```python
from build123d import *

# Parameters (mm, degrees)
PAD025_DEPTH    = 1
SKETCH038_W     = 8.1
SKETCH038_H     = 3.05
SKETCH038_W_2   = 3.05
SKETCH038_H_2   = 8.1
POCKET013_DEPTH = 0.5
POCKET014_DEPTH = 0.25
POCKET015_DEPTH = 0.25
SKETCH041_W     = 8
SKETCH041_H     = 3
SKETCH041_W_2   = 3
SKETCH041_H_2   = 8
PAD026_DEPTH    = 0.5


with BuildPart() as part:
    # Sketch037 (on Face2 of Binder012) → Pad025 (new body)
    with BuildSketch(Plane(origin=(0, 0, -13), x_dir=(1, 0, 0), z_dir=(0, 0, -1))):
        Polygon((75, -58.333333), (52, -58.333333), (40.686291501, -47.019624501), (2.352991501, -47.019624501), (2.352991501, -33.980341499), (13, -23.333333), (13, -5.333333), (78, -5.333333), (64.751288694, -18.582044306), (64.751288694, -40.582044306), align=None)
    extrude(amount=-PAD025_DEPTH)

    # Sketch038 (on Face11 of Pad025) → Pocket013 (cut)
    with BuildSketch(Plane(origin=(0, 0, -13), x_dir=(1, 0, 0), z_dir=(0, 0, -1))):
        with Locations((13.677991501, -45.494624501)):
            Rectangle(SKETCH038_W, SKETCH038_H)
        with Locations((32.686291501, -45.494624501)):
            Rectangle(SKETCH038_W, SKETCH038_H)
        with Locations((63.226288694, -29.582044306)):
            Rectangle(SKETCH038_W_2, SKETCH038_H_2)
        Polygon((74.6861389697, -8.6471940303), (68.9585740421, -14.3747589579), (66.8018983595, -12.2180832753), (72.5294632871, -6.4905183477), align=None)
        Polygon((67.475, -45.299650673), (71.525, -52.3144564437), (68.8836225185, -53.8394564437), (64.8336225185, -46.824650673), align=None)
        Polygon((49.2069282143, -55.5402612143), (43.4793632867, -49.8126962867), (45.6360389693, -47.6560206041), (51.3636038969, -53.3835855317), align=None)
        with Locations((59.5, -56.808333)):
            Rectangle(SKETCH038_W, SKETCH038_H)
    extrude(amount=-POCKET013_DEPTH, mode=Mode.SUBTRACT)

    # Sketch039 (on Face7 of Pocket013) → Pocket014 (cut)
    with BuildSketch(Plane.XY.offset(-12)):
        Polygon((2.352991501, 47.019624501), (2.352991501, 33.980341499), (13, 23.333333), (13, 5.333333), (78, 5.333333), (77.5, 5.833333), (13.5, 5.833333), (13.5, 23.5404397812), (2.852991501, 34.1874482802), (2.852991501, 47.019624501), align=None)
    extrude(amount=-POCKET014_DEPTH, mode=Mode.SUBTRACT)

    # Sketch040 (on Face7 of Pocket014) → Pocket015 (cut)
    with BuildSketch(Plane.XY.offset(-12)):
        Polygon((64.751288694, 19.2891510872), (60.5, 23.5404397812), (13.5, 23.5404397812), (13.5, 23.0404397812), (60.2928932188, 23.0404397812), (64.751288694, 18.582044306), align=None)
    extrude(amount=-POCKET015_DEPTH, mode=Mode.SUBTRACT)

    # Sketch041 (on Face2 of Pocket015) → Pad026 (join)
    with BuildSketch(Plane(origin=(0, 0, -13), x_dir=(1, 0, 0), z_dir=(0, 0, -1))):
        with Locations((68.5, -3.833333)):
            Rectangle(SKETCH041_W, SKETCH041_H)
        with Locations((45.5, -3.833333)):
            Rectangle(SKETCH041_W, SKETCH041_H)
        with Locations((22.5, -3.833333)):
            Rectangle(SKETCH041_W, SKETCH041_H)
        with Locations((11.5, -14.333333)):
            Rectangle(SKETCH041_W_2, SKETCH041_H_2)
        with Locations((0.852991501, -38.980341499)):
            Rectangle(SKETCH041_W_2, SKETCH041_H_2)
        Polygon((4.8278652352, -31.5054677648), (10.4847194847, -25.8486135153), (8.3633991411, -23.7272931718), (2.7065448916, -29.3841474213), align=None)
    extrude(amount=-PAD026_DEPTH)


solid = part.part
```
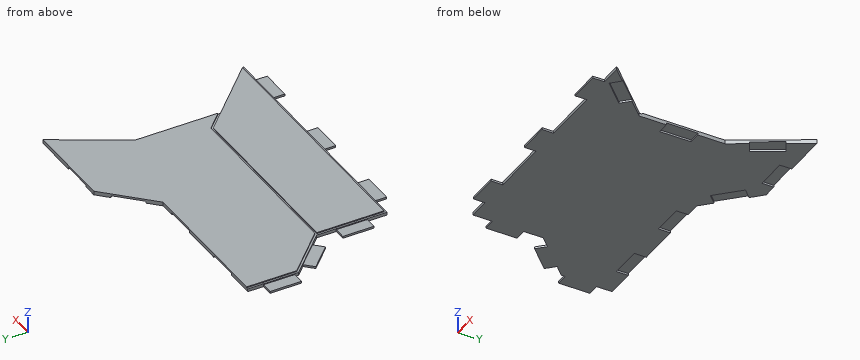
Build history of the part. All positions in model axes, mm. Give positions to 0.01 mm unless a question says otherwise; leave off trailing zeros. Order: outer loops, then holes, each group sorted by start corner. A loop starts at its lowest first (then second) coordinate and runs counter-clockwise, first axis right, second up. Notation, with made-up numbers: M 68.5,62 L 80.5,62 A27 ccw 80.5,100 Z; hole C 37,1 d4. An arc over 180 degrees is marked long. Return JSON: item names as keys, results as strings.
Q1. Band-saw the part on D-D (y = 51). Give the cut face in (x, z), then the cut area to 3 significant figures.
Answer list:
{"outline": "M 44.67,-12.5 L 48.98,-12.5 L 48.98,-13 L 67.24,-13 L 67.24,-12.5 L 70.77,-12.5 L 70.77,-12 L 44.67,-12 Z", "area": "22.2 mm^2"}
Q2. Wall check: probe 1 along Y at (x, z) = (36.5, -12.05); probe 2 along Y at (x, z) = (53, -12.35); probe 3 along Y at (x, z) = (73, -12.6). Give the ranges that are in metal, low to high. Write a range as from..to.
Answer list:
{"probe 1": "y = 5.83..23.04, 23.54..47.02", "probe 2": "y = 5.33..58.33", "probe 3": "y = 5.33..6.96, 54.87..58.33"}
Q3. Band-saw the part on C-C (y = 28). Give the cut face in (x, z), then the cut area to 3 significant figures.
Answer list:
{"outline": "M 4.09,-13 L 61.7,-13 L 61.7,-12.5 L 64.75,-12.5 L 64.75,-12 L 9.04,-12 L 9.04,-12.25 L 8.33,-12.25 L 8.33,-12.5 L 4.09,-12.5 Z", "area": "56.8 mm^2"}
Q4. Flat gauge pins, fed straight in: pin 1 (12 mm diameter, centred on x = 68, y = 19.5, fed in from +Z); pin 2 (0.9 mm diameter, centred on x = 23, y = 4.5, fed in from +Z); pin 3 (0.6 mm diameter, centred on y = 3.5, z = -12.5, fed in from -X); pin 4 (3.5 mm diameter, centred on x = 67.5, y = 4, fed in from +Z). Where does each tip first touch, or does it go through?
Answer list:
{"pin 1": "stops at z = -12", "pin 2": "stops at z = -12.5", "pin 3": "stops at x = 18.5", "pin 4": "stops at z = -12.25"}
Q5. Band-saw the part on B-B (y = 38). Give the cut face in (x, z), then the cut area to 3 significant figures.
Answer list:
{"outline": "M -0.65,-13 L 64.75,-13 L 64.75,-12 L 2.85,-12 L 2.85,-12.25 L 2.35,-12.25 L 2.35,-12.5 L -0.65,-12.5 Z", "area": "63.8 mm^2"}
Q6. Band-saw the part on A-A (x = 53). Give the cut face in (y, z), then the cut area to 4 significant figures.
Answer list:
{"outline": "M 5.33,-13 L 58.33,-13 L 58.33,-12 L 23.54,-12 L 23.54,-12.25 L 23.04,-12.25 L 23.04,-12 L 5.83,-12 L 5.83,-12.25 L 5.33,-12.25 Z", "area": "52.75 mm^2"}
